```python
from build123d import *

# Parameters (mm, degrees)
SKETCH1_W           = 105
SKETCH1_H           = 3
BOSS_EXTRUDE1_DEPTH = 300
SKETCH2_R           = 2
SKETCH2_R_2         = 1.374892706
SKETCH2_R_3         = 1.354217853
SKETCH2_R_4         = 1.307593734
SKETCH2_R_5         = 1.273931832
CUT_EXTRUDE1_DEPTH  = 10


with BuildPart() as part:
    # Sketch1 → Boss-Extrude1 (new body)
    with BuildSketch(Plane(origin=(0, 0, 0), x_dir=(0, 0, -1), z_dir=(1, 0, 0))):
        Rectangle(SKETCH1_W, SKETCH1_H)
    extrude(amount=-BOSS_EXTRUDE1_DEPTH)

    # Sketch2 → Cut-Extrude1 (cut)
    with BuildSketch(Plane.XZ.offset(1.5)):
        with Locations(Location((-187.17418267, 18.052570887, 0), (0, 0, 270))):
            Circle(SKETCH2_R)
        with Locations(Location((-157.57418267, 18.052570887, 0), (0, 0, 270))):
            Circle(SKETCH2_R)
        with Locations(Location((-157.57418267, 47.652570887, 0), (0, 0, 270))):
            Circle(SKETCH2_R)
        with Locations(Location((-187.17418267, 47.652570887, 0), (0, 0, 270))):
            Circle(SKETCH2_R)
        with Locations(Location((-203.080283558, 5.823951961, 0), (0, 0, 270))):
            Circle(SKETCH2_R_2)
        with Locations(Location((-146.289268611, 5.713822454, 0), (0, 0, 270))):
            Circle(SKETCH2_R_3)
        with Locations(Location((-146.435482331, -42.141729042, 0), (0, 0, 270))):
            Circle(SKETCH2_R_4)
        with Locations(Location((-203.080283558, -42.071168524, 0), (0, 0, 270))):
            Circle(SKETCH2_R_5)
        with Locations(Location((-157.57418267, -36.654156393, 0), (0, 0, 270))):
            Circle(SKETCH2_R)
        with Locations(Location((-187.17418267, -36.654156393, 0), (0, 0, 270))):
            Circle(SKETCH2_R)
        with Locations(Location((-216.77418267, -36.654156393, 0), (0, 0, 270))):
            Circle(SKETCH2_R)
        with Locations(Location((-91.671041898, 37.247626886, 0), (0, 0, 270))):
            Circle(SKETCH2_R)
        with Locations(Location((-216.77418267, 47.652570887, 0), (0, 0, 270))):
            Circle(SKETCH2_R)
        with Locations(Location((-254.388823597, 47.652570887, 0), (0, 0, 270))):
            Circle(SKETCH2_R)
        with Locations(Location((-275.97418267, 47.652570887, 0), (0, 0, 270))):
            Circle(SKETCH2_R)
        with Locations(Location((-157.57418267, -5.272741789, 0), (0, 0, 270))):
            Circle(SKETCH2_R)
        with Locations(Location((-187.17418267, -5.272741789, 0), (0, 0, 270))):
            Circle(SKETCH2_R)
        with Locations(Location((-216.77418267, -5.272741789, 0), (0, 0, 270))):
            Circle(SKETCH2_R)
        with Locations(Location((-232.313628015, 47.652570887, 0), (0, 0, 270))):
            Circle(SKETCH2_R)
        with Locations(Location((-275.97418267, -5.272741789, 0), (0, 0, 270))):
            Circle(SKETCH2_R)
        with Locations(Location((-275.97418267, -36.654156393, 0), (0, 0, 270))):
            Circle(SKETCH2_R)
        with Locations(Location((-232.313628015, -5.272741789, 0), (0, 0, 270))):
            Circle(SKETCH2_R)
        with Locations(Location((-232.313628015, 28.747940449, 0), (0, 0, 270))):
            Circle(SKETCH2_R)
        with Locations(Location((-254.388823597, 28.747940449, 0), (0, 0, 270))):
            Circle(SKETCH2_R)
        with Locations(Location((-254.388823597, -5.272741789, 0), (0, 0, 270))):
            Circle(SKETCH2_R)
        with Locations(Location((-254.388823597, -36.654156393, 0), (0, 0, 270))):
            Circle(SKETCH2_R)
        with Locations(Location((-232.313628015, -36.654156393, 0), (0, 0, 270))):
            Circle(SKETCH2_R)
        with Locations(Location((-53.671041898, 37.247626886, 0), (0, 0, 270))):
            Circle(SKETCH2_R)
        with Locations(Location((-15.671041898, 37.247626886, 0), (0, 0, 270))):
            Circle(SKETCH2_R)
        with Locations(Location((-129.671041898, 37.247626886, 0), (0, 0, 270))):
            Circle(SKETCH2_R)
        with Locations(Location((-129.671041898, 9.821730669, 0), (0, 0, 270))):
            Circle(SKETCH2_R)
        with Locations(Location((-91.671041898, 9.821730669, 0), (0, 0, 270))):
            Circle(SKETCH2_R)
        with Locations(Location((-53.671041898, 9.821730669, 0), (0, 0, 270))):
            Circle(SKETCH2_R)
        with Locations(Location((-15.671041898, 9.821730669, 0), (0, 0, 270))):
            Circle(SKETCH2_R)
        with Locations(Location((-129.671041898, -37.247626886, 0), (0, 0, 90))):
            Circle(SKETCH2_R)
        with Locations(Location((-129.671041898, -9.821730669, 0), (0, 0, 90))):
            Circle(SKETCH2_R)
        with Locations(Location((-91.671041898, -9.821730669, 0), (0, 0, 90))):
            Circle(SKETCH2_R)
        with Locations(Location((-53.671041898, -9.821730669, 0), (0, 0, 90))):
            Circle(SKETCH2_R)
        with Locations(Location((-15.671041898, -9.821730669, 0), (0, 0, 90))):
            Circle(SKETCH2_R)
        with Locations(Location((-91.671041898, -37.247626886, 0), (0, 0, 90))):
            Circle(SKETCH2_R)
        with Locations(Location((-53.671041898, -37.247626886, 0), (0, 0, 90))):
            Circle(SKETCH2_R)
        with Locations(Location((-15.671041898, -37.247626886, 0), (0, 0, 90))):
            Circle(SKETCH2_R)
        with BuildLine():
            Line((-9.819471051, -34.403955007), (-9.819471051, -15.203651424))
            ThreePointArc((-9.819471051, -15.203651424), (-7.18680013, -12.570980503), (-4.554129209, -15.203651424))
            Line((-4.554129209, -15.203651424), (-4.554129209, -34.403955007))
            ThreePointArc((-4.554129209, -34.403955007), (-7.18680013, -37.036625928), (-9.819471051, -34.403955007))
        make_face()
        with BuildLine():
            Line((-4.430775444, 33.91650296), (-4.430775444, 15.317539102))
            ThreePointArc((-4.430775444, 15.317539102), (-7.18680013, 12.561514417), (-9.942824816, 15.317539102))
            Line((-9.942824816, 15.317539102), (-9.942824816, 33.91650296))
            ThreePointArc((-9.942824816, 33.91650296), (-7.18680013, 36.672527645), (-4.430775444, 33.91650296))
        make_face()
    extrude(amount=-CUT_EXTRUDE1_DEPTH, mode=Mode.SUBTRACT)


solid = part.part
```
Can you work these out from the model? Positions are in its coordinate system, mm. Coordinates: 2 decimals unless noted, no trailing zeros. Loops run counter-clockwise (first coordinate to the right, second up) from the corner with the lowest first, then second, coordinate; pieces in that order, holes last. Notation, with made-up numbers: M -33.5,57.5 L -9.5,57.5 A15 cw -9.5,73.5 Z; hole C 77.25,-23.75 d2. An arc over 180 degrees is marked long. Put each result on its own line as item: value. Start each with the question number.
(1) Imagine slicing it at B-B on y = -0.95. Give the number of separate pieces and of enclosed holes in the cut face, and give its area (3 significant figures).
(2) I need wall thicknesses on probe 1 along Z at (x, y) = (-92, -0.95); probe 2 along X at (y, z) = (0.2, 15.5); probe 3 along X at (y, z) = (-0.95, -34). Which ranges of each line are inside material? Lowest first, please.
(3) Imagine slicing it at A-A on z = -21. List the corners of the cut face in (x, y) for me, and give its area (3 significant figures).
Worked answers:
1. separate pieces: 1
1. enclosed holes: 44
1. area: 30,800 mm2
2. probe 1: z = -52.5 to -39.22, -35.27 to -11.79, -7.85 to 7.85, 11.79 to 35.27, 39.22 to 52.5
2. probe 2: x = -300 to -9.94, -4.43 to 0
2. probe 3: x = -300 to -9.82, -4.55 to 0
3. outline: M -300,-1.5 L -9.82,-1.5 L -9.82,1.5 L -300,1.5 Z; M -4.55,-1.5 L 0,-1.5 L 0,1.5 L -4.55,1.5 Z
3. area: 884 mm2
